Design review of the part shown in the three views and the two pictorial views. Dimensions are in mm from the part's minimum x, y and z. A direction names the side the tool comes from. Round coordinates to 2 decimals unless told otherwise and drop trailing zeros. Order: outer loops, then holes, each group sorted by start corner. A loop starts at its lowest first (then second) coordinate and runs counter-clockwise, first axis right, second up.
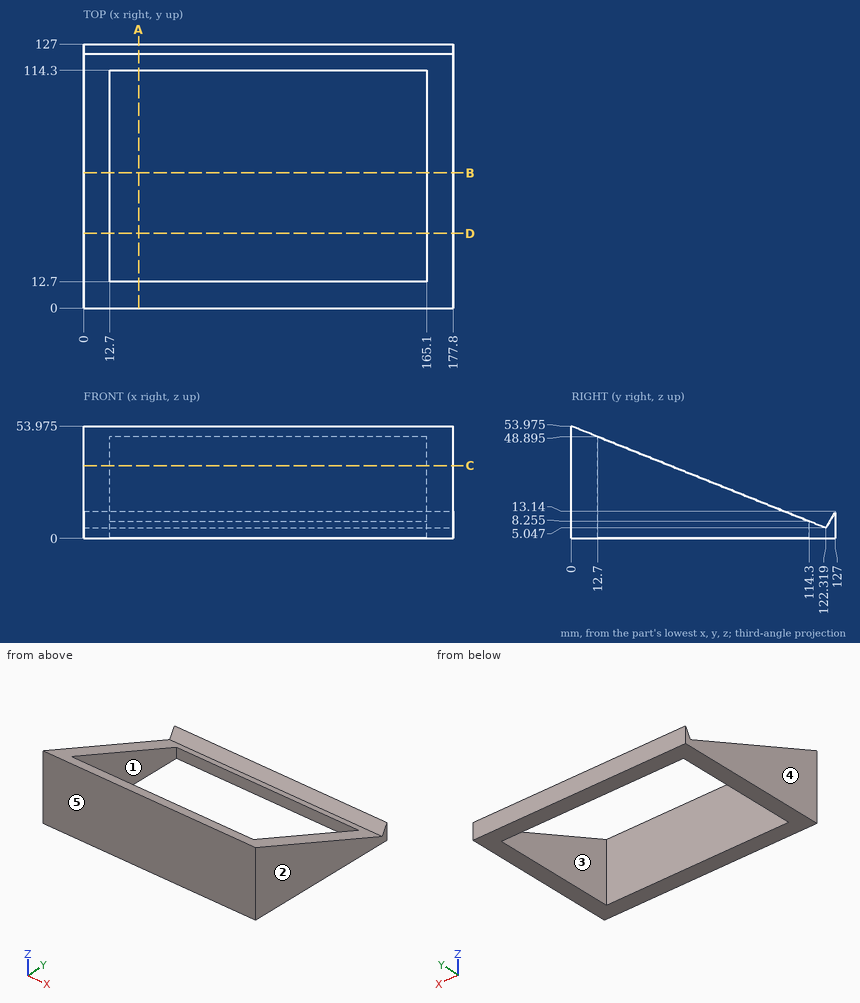
1) To check wall thickness, follow line 1 along X through (y, z) = (57.5, 18); line 2 along Y through (x, z) = (62, 29); line 3 along Z through (x, y) = (138.5, 117) (1 decimal). State the ranges of each line that lie inside material, in increasing order.
Results:
line 1: x = 0 to 12.7, 165.1 to 177.8
line 2: y = 0 to 12.7
line 3: z = 0 to 7.2
2) Take a section at C-C on z = 35. Give the boundary of the cut face in (x, y), plus the area to 3 significant figures.
Results:
outline: (0, 0) - (177.8, 0) - (177.8, 47.44) - (165.1, 47.44) - (165.1, 12.7) - (12.7, 12.7) - (12.7, 47.44) - (0, 47.44) - close
area: 3,140 mm2
3) For the marked faces 1 and 2, list the 3-axis set-ups (+Z, -Z, +X, -X, +Y, -Y) from which the entire face can be reached by the end or side of a thin tool; tool diameter is ignored.
Results:
face 1: +Z, -Z
face 2: +Z, -Z, +X, +Y, -Y
4) The part is to be moulded in two halves that separate along Y. For the marked faces 3, 4 and 5, say which applies: released by +Y, released by -Y, zero draft, split by the parting line, or undercut.
Results:
face 3: undercut
face 4: zero draft
face 5: released by -Y
5) Take a section at A-A on x = 26.5. Give the boundary of the cut face in (y, z) (1 decimal).
Results:
outline: (0, 0) - (12.7, 0) - (12.7, 48.9) - (0, 54) - close; (114.3, 0) - (127, 0) - (127, 13.1) - (122.3, 5) - (114.3, 8.3) - close
6) Take a section at D-D on y = 36. Give the boundary of the cut face in (x, z) (1 decimal).
Results:
outline: (0, 0) - (12.7, 0) - (12.7, 39.6) - (0, 39.6) - close; (165.1, 0) - (177.8, 0) - (177.8, 39.6) - (165.1, 39.6) - close
7) Take a section at B-B on y = 65. Give the boundary of the cut face in (x, z) (1 decimal).
Results:
outline: (0, 0) - (12.7, 0) - (12.7, 28) - (0, 28) - close; (165.1, 0) - (177.8, 0) - (177.8, 28) - (165.1, 28) - close
8) Clearance check with a flat-ended pin moving along its axis: P1, Ø12, axis at x = 113, z = 24, coming from the +Y side. State where the tip first meets the part, or that it passes through.
Results:
P1: stops at y = 12.7
